from build123d import *

# Parameters (mm, degrees)
F0_W     = 120.904
F0_H     = 57.404
F1_DEPTH = 26.924
F2_W     = 66.548
F2_H     = 17.78
F3_DEPTH = 53.849
F5_DEPTH = 53.849
F6_W     = 28.448
F6_H     = 14.224
F7_DEPTH = 57.405
F9_DEPTH = 57.405


with BuildPart() as f1:
    # F0 (on Front) → F1 (new body, symmetric)
    with BuildSketch(Plane.XZ):
        with Locations((60.452, 28.702)):
            Rectangle(F0_W, F0_H)
    extrude(amount=F1_DEPTH, both=True)

    # F2 (on face) → F3 (cut, through all)
    with BuildSketch(Plane.XZ.offset(26.924)):
        with Locations((33.274, 8.89)):
            Rectangle(F2_W, F2_H)
    extrude(amount=-F3_DEPTH, mode=Mode.SUBTRACT)

    # F4 (on face) → F5 (cut, through all)
    with BuildSketch(Plane.XZ.offset(26.924)):
        Polygon((120.904, 28.702), (120.904, 57.404), (71.190678, 57.404), align=None)
    extrude(amount=-F5_DEPTH, mode=Mode.SUBTRACT)

    # F6 (on face) → F7 (cut, through all)
    with BuildSketch(Plane.XY.offset(57.404)):
        with Locations((106.68, -19.812)):
            Rectangle(F6_W, F6_H)
        with Locations((106.68, 19.812)):
            Rectangle(F6_W, F6_H)
    extrude(amount=-F7_DEPTH, mode=Mode.SUBTRACT)

    # F8 (on face) → F9 (cut, through all)
    with BuildSketch(Plane.XY.offset(57.404)):
        with BuildLine():
            Line((44.704, 7.874), (19.304, 7.874))
            ThreePointArc((19.304, 7.874), (11.43, 0), (19.304, -7.874))
            Line((19.304, -7.874), (44.704, -7.874))
            ThreePointArc((44.704, -7.874), (52.578, 0), (44.704, 7.874))
        make_face()
    extrude(amount=-F9_DEPTH, mode=Mode.SUBTRACT)


solid = f1.part
Here's how the part is built. I have some questions about the finished solid (model axes, mm). A direction names the side the tool comes from. Give positions to 0.01 mm unless a question says otherwise; leave off trailing zeros. Loops run counter-clockwise (first coordinate to the right, second up) from the corner with the lowest first, then second, coordinate; pieces in that order, holes last. Notation, with made-up numbers: (12, 8.5) -> (18, 8.5) arc R23 cw to (18, 47.5) -> close; hole circle Ø7 at (27, 49). An arc over 180 degrees is marked (long way). One line per item, written item: value.
Q1. I'm going to push flat-ended pins straight in: pin 1 Ø14 at (x, z) = (104.5, 23.5) entering from +Y; pin 2 Ø2 at (x, y) = (28, -12) entering from -Z; pin 3 Ø8 at (x, y) = (79.5, 19.5) entering from +Z. Where does each tip first touch, or does it pass through?
Answers follow:
pin 1: y = 12.7
pin 2: z = 17.78
pin 3: z = 54.92
Q2. Suppose I cut it at C-C on z = 24.5. Please give me the cut outline in (x, y).
Answers follow:
outline: (0, -26.92) -> (92.46, -26.92) -> (92.46, -12.7) -> (120.9, -12.7) -> (120.9, 12.7) -> (92.46, 12.7) -> (92.46, 26.92) -> (0, 26.92) -> close; hole (19.3, -7.87) -> (44.7, -7.87) arc R7.87 ccw to (44.7, 7.87) -> (19.3, 7.87) arc R7.87 ccw to start
Q3. On a 3-axis mill with a long thin cutter (end or side, diameter ignored), from which of +Z, -Z, +X, -X, +Y, -Y can I reach the whole of each face in a straight line? I mean faces 5 (the face through (52.576, -0.173, 37.869)), 6 (the face through (0, 0, 37)), 7 (the face through (106, 12.7, 18)), 8 (the face through (33, -12, 17.78)), 9 (the face through (92.456, -20, 23)). Say none if no direction works.
Answers follow:
face 5: +Z, -Z
face 6: +Z, -Z, -X, +Y, -Y
face 7: +Z, -Z, +X, +Y
face 8: -Z, -X, +Y, -Y
face 9: +Z, -Z, +X, -Y
Q4. If I drill on line 1 along Y through (x, z) = (33.5, 41.5); line 2 along Z through (x, y) = (7, 13); line 3 along X through (y, z) = (-18, 26.5), over which ranges is the centre line in solid material (lowest first)?
Answers follow:
line 1: -26.92 to -7.87, 7.87 to 26.92
line 2: 17.78 to 57.4
line 3: 0 to 92.46
Q5. We'd pull the mould along X, two halves only. Please class faces 1 (the face through (46, 26.924, 35)), 2 (the face through (32, 7.874, 38)), 3 (the face through (32, -7.874, 38)), 4 (the face through (66.548, 0, 9)): pulls with the +X half, pulls with the -X half, needs draft (parallel to the pull), parting line crosses it, or undercut.
Answers follow:
face 1: needs draft
face 2: undercut
face 3: undercut
face 4: pulls with the -X half
Q6. Suppose I cut it at B-B on y = 0. Please give me the cut outline in (x, z).
Answers follow:
outline: (0, 17.78) -> (11.43, 17.78) -> (11.43, 57.4) -> (0, 57.4) -> close; (52.58, 17.78) -> (66.55, 17.78) -> (66.55, 0) -> (120.9, 0) -> (120.9, 28.7) -> (71.19, 57.4) -> (52.58, 57.4) -> close
Q7. Suppose I cut it at D-D on y = -21. Please give me the cut outline in (x, z), then the cut area to 3 significant figures.
Answers follow:
outline: (0, 17.78) -> (66.55, 17.78) -> (66.55, 0) -> (92.46, 0) -> (92.46, 45.13) -> (71.19, 57.4) -> (0, 57.4) -> close
area: 3,990 mm^2
Q8. Suppose I cut it at A-A on x = 32. Please give me the cut outline in (y, z).
Answers follow:
outline: (-26.92, 17.78) -> (-7.87, 17.78) -> (-7.87, 57.4) -> (-26.92, 57.4) -> close; (7.87, 17.78) -> (26.92, 17.78) -> (26.92, 57.4) -> (7.87, 57.4) -> close
